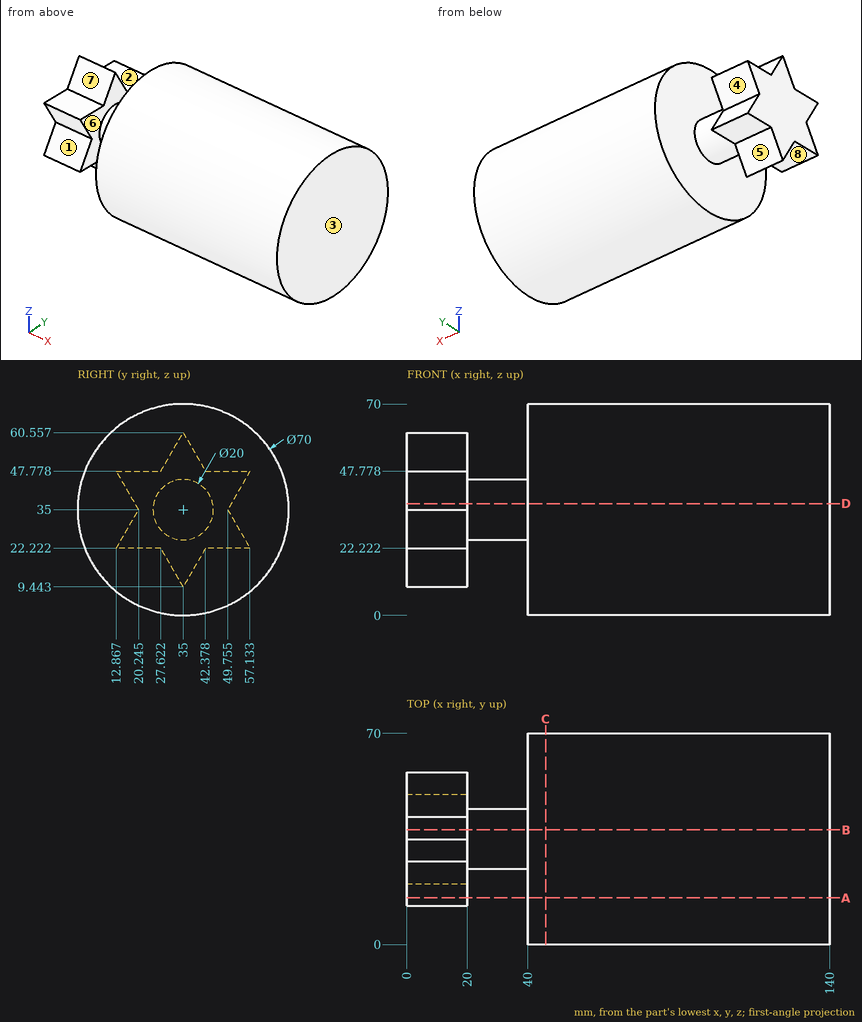
For this review, use the dimensioned drawing (mm, ordinates from the lowest corner) and the shaded views. A direction names the side the tool comes from. Coordinates: 2 decimals unless noted, no trailing zeros. Loops run counter-clockwise (first coordinate to the right, second up) from the corner with the lowest first, then second, coordinate; pieces in that order, holes last. Notation, with made-up numbers: (39, 51) - (71, 51) arc R23 cw to (71, 90) - close; hole circle Ø10 at (19.25, 6.5). An arc over 180 degrees is marked (long way). Use one line per item in the form item = value. Start each with the question number.
1) For the marked faces 4, 5, 6, 7 and 8, list the 3-axis set-ups (+Z, -Z, +X, -X, +Y, -Y) from which the entire face can be reached by the end or side of a thin tool; tool diameter is ignored.
2) For pin 1 (16 mm diameter, centred on x = 5.5, y = 52, fed in from +Z); pin 2 (7.5 mm diameter, centred on x = 11, y = 22, fed in from -Z); pin 3 (12 mm diameter, centred on x = 57, y = 36.5, fed in from -Z); pin 4 (4 mm diameter, centred on y = 43.5, z = 24, fed in from -X), all flat-tipped, find the tip position at first contact; note any pin that passes through.
3) Draft analysis for pull direction Z (two halves, no side actions). For the marked faces 1, 2 and 3, state which applies: released by +Z, released by -Z, zero draft, split by the parting line, or undercut.
4) Take a section at C-C (x = 46). State the section outline as (y, z) points, plus the area to 3 significant figures.
5) To check wall thickness, follow probe 1 along X at (y, z) = (42.5, 24); probe 2 along X at (y, z) = (58, 17.5); probe 3 along Z at (x, y) = (9, 53) (1 decimal). State the ranges of each line that lie inside material, in increasing order. Write a range as from..to.
6) Take a section at B-B (y = 38). State the section outline as (x, z) points, plus the area to 3 significant figures.
7) Take a section at D-D (z = 37). State the section outline as (x, y) points.
8) Take a section at A-A (y = 15.5). State the section outline as (x, z) points (1 decimal).
From the geometry:
q1.face_4 = -X, +Y
q1.face_5 = -Z, -X, +Y
q1.face_6 = none
q1.face_7 = +Z, -X, -Y
q1.face_8 = -Z, -X, -Y
q2.pin_1 = 47.78
q2.pin_2 = 22.22
q2.pin_3 = 0
q2.pin_4 = 0
q3.face_1 = undercut
q3.face_2 = released by +Z
q3.face_3 = zero draft
q4.outline = circle Ø70 at (35, 35)
q4.area = 3,850 mm2
q5.probe_1 = 0..20, 40..140
q5.probe_2 = 40..140
q5.probe_3 = 22.2..29.4, 40.6..47.8
q6.outline = (0, 14.64) - (20, 14.64) - (20, 25.46) - (40, 25.46) - (40, 0.13) - (140, 0.13) - (140, 69.87) - (40, 69.87) - (40, 44.54) - (20, 44.54) - (20, 55.36) - (0, 55.36) - close
q6.area = 8,170 mm2
q7.outline = (0, 19.09) - (20, 19.09) - (20, 25.2) - (40, 25.2) - (40, 0.06) - (140, 0.06) - (140, 69.94) - (40, 69.94) - (40, 44.8) - (20, 44.8) - (20, 50.91) - (0, 50.91) - close
q8.outline = (0, 22.2) - (20, 22.2) - (20, 26.8) - (0, 26.8) - close; (0, 43.2) - (20, 43.2) - (20, 47.8) - (0, 47.8) - close; (40, 5.9) - (140, 5.9) - (140, 64.1) - (40, 64.1) - close
